Can you work these out from the model? Positions are in its coordinate system, mm. A direction names the side the tool comes from. Coordinates: 2 decimals unless noted, no trailing zeros. Loops run counter-clockwise (first coordinate to the right, second up) from the corner with the lowest first, then second, coordinate; pieces in that order, holes last. Notation, with made-up numbers: (64.5, -22) -> (103.5, -22) arc R11 cw to (103.5, -18) -> close; hole circle Ø1 at (72, 88.5). An arc over 180 degrees is marked (long way). Use one line per item in the form item = value. Start each with the question number.
(1) On a 3-axis mill with a long thin cutter (end or side, diameter ignored), from which of +Z, -Z, +X, -X, +Y, -Y can I reach the whole of each face in a straight line? I mean faces 1 (the flat face through (-7, 1.842, 8)), 2 (the flat face through (-7, 1, 54.928)). Say none if no direction works.
(2) Imagine slicing it at D-D (x = -11.5). List the corners of the cut face in (y, z) for me, plus the area to 3 significant figures.
(3) I'm going to push flat-ended pins straight in: pin 1 (4 mm diameter, centred on x = -9.5, z = 34, fed in from +Y); pin 2 (0.6 mm diameter, centred on y = 1.5, z = 40, fed in from +X). Where does each tip first touch, or does it pass through?
(4) Imagine slicing it at B-B (x = -6.5). List the corners of the cut face in (y, z) for me, plus the area to 3 significant figures.
(5) Imagine slicing it at A-A (y = 0.7). List the corners of the cut face in (x, z) for me, plus the area to 3 significant figures.
(6) Thinking about a two-plate mould opening in Z: for faces 3 (the flat face through (-6, 0, 42)), 4 (the flat face through (-7, 1, 76.2)), 5 (the flat face through (-7, 1, 26.67)), 6 (the flat face through (-7, 1, 5.398)), which applies, released by +Z, released by -Z, zero draft, split by the parting line, or undercut?
(7) I need wall thicknesses on line 1 (Z direction, x = -4.25, y = 0.3); line 2 (Y direction, x = -7.75, z = 11); line 3 (X direction, y = 1.4, z = 6) (1 decimal). Which ranges of each line are inside material? Lowest first, please. Write a range as [from, to].
Autodesk Inventor part; units mm, degrees
ref_plane "YZ Plane" through (0, 0, 0) normal (1, 0, 0) x (0, 1, 0)
ref_plane "XZ Plane" through (0, 0, 0) normal (0, 1, 0) x (-1, 0, 0)
ref_plane "XY Plane" through (0, 0, 0) normal (0, 0, 1) x (1, 0, 0)
sketch "Sketch1" plane through (0, 0, 0) normal (0, 1, 0) x (-1, 0, 0)
  line L0 (0, 0) -> (12.7, 0)
  line L1 (12.7, 0) -> (12.7, 82.55)
  line L2 (12.7, 82.55) -> (0, 82.55)
  line L3 (0, 82.55) -> (0, 0)
  dimension "d0" = 12.7
  dimension "d1" = 82.55
extrude "Extrusion1" add sketch "Sketch1" along normal blind 0.254
sketch "Sketch2" plane through (0, 0.254, 0) normal (0, 1, 0) x (1, 0, 0)
  line L0 (-9.525, -76.2) -> (-4.7625, -76.2)
  line L1 (-4.7625, -76.2) -> (-4.7625, -71.4375)
  line L2 (-4.7625, -71.4375) -> (-9.525, -71.4375)
  line L3 (-9.525, -71.4375) -> (-9.525, -76.2)
  line L4 (-12.7, -82.55) -> (0, -82.55)
  line L5 (-12.7, 0) -> (-12.7, -82.55)
  line L6 (-9.525, -59.69) -> (-4.7625, -59.69)
  line L7 (-4.7625, -59.69) -> (-4.7625, -54.9275)
  line L8 (-4.7625, -54.9275) -> (-9.525, -54.9275)
  line L9 (-9.525, -54.9275) -> (-9.525, -59.69)
  line L10 (-9.525, -43.18) -> (-4.7625, -43.18)
  line L11 (-4.7625, -43.18) -> (-4.7625, -38.4175)
  line L12 (-4.7625, -38.4175) -> (-9.525, -38.4175)
  line L13 (-9.525, -38.4175) -> (-9.525, -43.18)
  line L14 (-9.525, -26.67) -> (-4.7625, -26.67)
  line L15 (-4.7625, -26.67) -> (-4.7625, -21.9075)
  line L16 (-4.7625, -21.9075) -> (-9.525, -21.9075)
  line L17 (-9.525, -21.9075) -> (-9.525, -26.67)
  line L18 (-9.525, -10.16) -> (-4.7625, -10.16)
  line L19 (-4.7625, -10.16) -> (-4.7625, -5.3975)
  line L20 (-4.7625, -5.3975) -> (-9.525, -5.3975)
  line L21 (-9.525, -5.3975) -> (-9.525, -10.16)
  line L22 (-4.7625, -59.69) -> (-3.7465, -59.69)
  line L23 (-3.7465, -59.69) -> (-3.7465, -54.9275)
  line L24 (-3.7465, -54.9275) -> (-4.7625, -54.9275)
  line L25 (-4.7625, -54.9275) -> (-4.7625, -59.69)
  line L26 (-4.7625, -76.2) -> (-3.7465, -76.2)
  line L27 (-3.7465, -76.2) -> (-3.7465, -71.4375)
  line L28 (-3.7465, -71.4375) -> (-4.7625, -71.4375)
  line L29 (-4.7625, -71.4375) -> (-4.7625, -76.2)
  line L30 (-9.525, -76.2) -> (-10.541, -76.2)
  line L31 (-10.541, -76.2) -> (-10.541, -71.4375)
  line L32 (-10.541, -71.4375) -> (-9.525, -71.4375)
  line L33 (-9.525, -71.4375) -> (-9.525, -76.2)
  line L34 (-9.525, -59.69) -> (-10.541, -59.69)
  line L35 (-10.541, -59.69) -> (-10.541, -54.9275)
  line L36 (-10.541, -54.9275) -> (-9.525, -54.9275)
  line L37 (-9.525, -54.9275) -> (-9.525, -59.69)
  line L38 (-9.525, -43.18) -> (-10.541, -43.18)
  line L39 (-10.541, -43.18) -> (-10.541, -38.4175)
  line L40 (-10.541, -38.4175) -> (-9.525, -38.4175)
  line L41 (-9.525, -38.4175) -> (-9.525, -43.18)
  line L42 (-4.7625, -43.18) -> (-3.7465, -43.18)
  line L43 (-3.7465, -43.18) -> (-3.7465, -38.4175)
  line L44 (-3.7465, -38.4175) -> (-4.7625, -38.4175)
  line L45 (-4.7625, -38.4175) -> (-4.7625, -43.18)
  line L46 (-4.7625, -26.67) -> (-3.7465, -26.67)
  line L47 (-3.7465, -26.67) -> (-3.7465, -21.9075)
  line L48 (-3.7465, -21.9075) -> (-4.7625, -21.9075)
  line L49 (-4.7625, -21.9075) -> (-4.7625, -26.67)
  line L50 (-9.525, -26.67) -> (-10.541, -26.67)
  line L51 (-10.541, -26.67) -> (-10.541, -21.9075)
  line L52 (-10.541, -21.9075) -> (-9.525, -21.9075)
  line L53 (-9.525, -21.9075) -> (-9.525, -26.67)
  line L54 (-9.525, -10.16) -> (-10.541, -10.16)
  line L55 (-10.541, -10.16) -> (-10.541, -5.3975)
  line L56 (-10.541, -5.3975) -> (-9.525, -5.3975)
  line L57 (-9.525, -5.3975) -> (-9.525, -10.16)
  line L58 (-4.7625, -10.16) -> (-3.7465, -10.16)
  line L59 (-3.7465, -10.16) -> (-3.7465, -5.3975)
  line L60 (-3.7465, -5.3975) -> (-4.7625, -5.3975)
  line L61 (-4.7625, -5.3975) -> (-4.7625, -10.16)
  point P0 (0, 0)
  point P1 (-4.7625, -21.9075)
  point P2 (-4.7625, -54.9275)
  dimension "d4" = 4.7625
  dimension "d5" = 4.7625
  dimension "d6" = 6.35
  dimension "d7" = 3.175
  dimension "d8" = 4.7625
  dimension "d9" = 4.7625
  dimension "d10" = 11.7475
  dimension "d11" = 3.175
  dimension "d12" = 4.7625
  dimension "d13" = 4.7625
  dimension "d14" = 4.7625
  dimension "d15" = 4.7625
  dimension "d16" = 4.7625
  dimension "d17" = 4.7625
  dimension "d18" = 11.7475
  dimension "d19" = 11.7475
  dimension "d20" = 11.7475
  dimension "d21" = 3.175
  dimension "d22" = 1.016
  dimension "d23" = 1.016
  dimension "d31" = 4.7625
  dimension "d32" = 4.7625
  dimension "d33" = 4.7625
  dimension "d34" = 4.7625
extrude "Extrusion2" add sketch "Sketch2" along normal blind 1.5875 contours L3 L2 L1 L0 | L9 L8 L7 L6 | L13 L12 L11 L10 | L17 L16 L15 L14 | L21 L20 L19 L18
extrude "Extrusion3" add sketch "Sketch2" along normal blind 0.7937 contours L30 L31 L32 L3 | L1 L28 L27 L26 | L34 L35 L36 L9 | L7 L24 L23 L22 | L38 L39 L40 L13 | L11 L44 L43 L42 | L50 L51 L52 L17 | L15 L48 L47 L46 | L54 L55 L56 L21 | L19 L60 L59 L58
chamfer "Chamfer1" distance 0.7937 angle 45 10 edges at (-3.7465, 1.0477, 73.8188) (-3.7465, 1.0477, 57.3088) (-3.7465, 1.0477, 40.7988) (-3.7465, 1.0477, 24.2888) (-3.7465, 1.0477, 7.7787) (-10.541, 1.0477, 7.7787) (-10.541, 1.0477, 24.2888) (-10.541, 1.0477, 40.7988) (-10.541, 1.0477, 57.3088) (-10.541, 1.0477, 73.8188)
properties part number "LED_Strip"
Worked out:
q1.face_1 = +Z, -Z, +X, -X, +Y
q1.face_2 = +X, -X, +Y
q2.outline = (0, 0) -> (0.25, 0) -> (0.25, 82.55) -> (0, 82.55) -> close
q2.area = 21.0 mm2
q3.pin_1 = 0.25
q3.pin_2 = -4.76
q4.outline = (0, 0) -> (0.25, 0) -> (0.25, 5.4) -> (1.84, 5.4) -> (1.84, 10.16) -> (0.25, 10.16) -> (0.25, 21.91) -> (1.84, 21.91) -> (1.84, 26.67) -> (0.25, 26.67) -> (0.25, 38.42) -> (1.84, 38.42) -> (1.84, 43.18) -> (0.25, 43.18) -> (0.25, 54.93) -> (1.84, 54.93) -> (1.84, 59.69) -> (0.25, 59.69) -> (0.25, 71.44) -> (1.84, 71.44) -> (1.84, 76.2) -> (0.25, 76.2) -> (0.25, 82.55) -> (0, 82.55) -> close
q4.area = 58.8 mm2
q5.outline = (-10.1, 5.4) -> (-4.19, 5.4) -> (-4.19, 10.16) -> (-10.1, 10.16) -> close; (-10.1, 21.91) -> (-4.19, 21.91) -> (-4.19, 26.67) -> (-10.1, 26.67) -> close; (-10.1, 38.42) -> (-4.19, 38.42) -> (-4.19, 43.18) -> (-10.1, 43.18) -> close; (-10.1, 54.93) -> (-4.19, 54.93) -> (-4.19, 59.69) -> (-10.1, 59.69) -> close; (-10.1, 71.44) -> (-4.19, 71.44) -> (-4.19, 76.2) -> (-10.1, 76.2) -> close
q5.area = 141 mm2
q6.face_3 = zero draft
q6.face_4 = released by +Z
q6.face_5 = undercut
q6.face_6 = released by -Z
q7.line_1 = [5.4, 10.16], [21.91, 26.67], [38.42, 43.18], [54.93, 59.69], [71.44, 76.2]
q7.line_2 = [0, 0.25]
q7.line_3 = [-9.5, -4.8]
